Verification items for the finished model (mm, model axes). Give positions to 0.01 mm unless a question says otherwise; leave off trailing zeros. Order: outer loops, then holes, each group sorted by start corner. A loop starts at its lowest first (then second) coordinate and runs counter-clockwise, first axis right, second up. Notation, with made-up numbers: (17.25, -20.75) -> (65.25, -20.75) arc R25 cw to (65.25, -7.75) -> close; hole circle Ø2 at (19.5, 20). An arc over 180 degrees is marked (long way). Return JSON: item names as keys, results as strings. Group by question number.
(1) Thickness scan on line 1 along X through (y, z) = (0, -7.75); line 2 along Z through (x, y) = (9, -71). Record the ranges inside material, lowest first.
(2) Depth check by flat-ended pin: pin 1 Ø8 at (y, z) = (-1, -15) entering from +X; pin 2 Ø5 at (x, z) = (-12, -19.5) entering from -Y; pin 3 Ø10 at (x, y) = (-25, -2) entering from -Z. Enter the tip coordinate at first touch or a pass-through.
(3) Cross-section at A-A on x = 0. Enter the section's corners in (y, z).
(4) Cross-section at B-B on z = -17. Enter the section's corners in (x, y), then the cut area to 3 significant figures.
(5) Release check for a two-part mould opening along X. For faces 1 (the face through (-0.59, -4.46, -15.8)), 2 (the face through (-2.38, 10.74, -14.79)), 3 (the face through (19, -4, 3)) record: pulls with the +X half, pulls with the -X half, needs draft (parallel to the pull), parting line crosses it, or undercut.
from build123d import *

# Parameters (mm, degrees)
F0_R     = 94.9025273368
F0_R_2   = 4.5
F1_DEPTH = 3
F2_R     = 11
F2_R_2   = 4.5
F3_DEPTH = 30


# Not quite as in the source:
# - a fillet or chamfer that OpenCascade refuses, or shapes differently, is made with other operations: its cross-section is extruded or revolved along the edge and cut away or added


with BuildPart() as f1:
    # F0 (on Top) → F1 (new body)
    with BuildSketch(Plane.XY):
        with Locations((0, -5.2974726632)):
            Circle(F0_R)
        Circle(F0_R_2, mode=Mode.SUBTRACT)
    extrude(amount=F1_DEPTH)

    # F2 (on face) → F3 (join)
    with BuildSketch(Plane(origin=(0, 0, 0), x_dir=(1, 0, 0), z_dir=(0, 0, -1))):
        Circle(F2_R)
        Circle(F2_R_2, mode=Mode.SUBTRACT)
    extrude(amount=F3_DEPTH)

    # F4: fillet of radius 5 on 2 edges, made by hand

    # F4_s1 → F4_t2 (revolve, cut)
    with BuildSketch(Plane.XZ.offset(5.2974726632)):
        with BuildLine():
            ThreePointArc((94.9025273368, 0), (93.0585644294, 2.1833001327), (90.3199516419, 3))
            Line((90.3199516419, 3), (94.9025273368, 3))
            Line((94.9025273368, 3), (94.9025273368, 0))
        make_face()
    revolve(axis=Axis((0, -5.2974726632, 3), (0, 0, 1)), mode=Mode.SUBTRACT)

    # F4_s3 → F4_t4 (revolve, cut)
    with BuildSketch(Plane.XZ):
        with BuildLine():
            ThreePointArc((9.5, 3), (5.9644660941, 1.5355339059), (4.5, -2))
            Line((4.5, -2), (4.5, 3))
            Line((4.5, 3), (9.5, 3))
        make_face()
    revolve(axis=Axis((0, 0, 3), (0, 0, 1)), mode=Mode.SUBTRACT)


solid = f1.part
Verdict:
{
 "1": {"line 1": "-11 to -4.5, 4.5 to 11", "line 2": "0 to 3"},
 "2": {"pin 1": "x = 11", "pin 2": "y = -5.55", "pin 3": "z = 0"},
 "3": {"outline": "(-100.2, 0) -> (-11, 0) -> (-11, -30) -> (-4.5, -30) -> (-4.5, -2) arc R5 ccw to (-9.5, 3) -> (-95.62, 3) arc R5 ccw to start; (4.5, -30) -> (11, -30) -> (11, 0) -> (89.61, 0) arc R5 ccw to (85.02, 3) -> (9.5, 3) arc R5 ccw to (4.5, -2) -> close"},
 "4": {"outline": "circle Ø22 at (0, 0); hole circle Ø9 at (0, 0)", "area": "317 mm²"},
 "5": {"face 1": "undercut", "face 2": "parting line crosses it", "face 3": "needs draft"}
}
